CAD build for the part. Positions are in the model's coordinates, mm. Face numbers are marked on the shaded views. A direction names the side the tool comes from. Round coordinates to 2 decimals unless told otherwise and drop trailing zeros. Loops run counter-clockwise (first coordinate to the right, second up) from the corner with the lowest first, then second, coordinate; pieces in that order, holes last. Notation, with made-up numbers: (28.5, -6) -> (74.5, -6) arc R32 cw to (74.5, 26) -> close; hole circle Ø5 at (88, 38.25). An arc over 180 degrees is marked (long way). Answer as CSV lines item,"result".
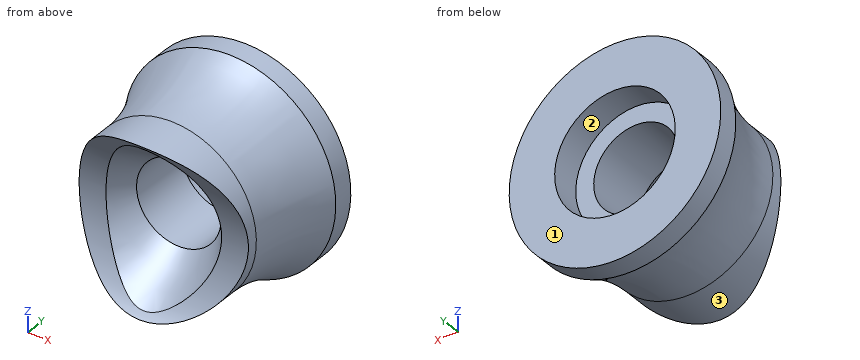
```python
from build123d import *

# Parameters (mm, degrees)
ENL_V_MAT_EXTRU_1_DEPTH      = 26
ENL_V_MAT_EXTRU_1_DEPTH_BACK = 26


with BuildPart() as part:
    # Esquisse1 → Révolution1 (revolve)
    with BuildSketch(Plane.XY, mode=Mode.PRIVATE) as r_volution1_sk:
        with BuildLine():
            Line((10, -22), (10, -7))
            Line((10, -7), (14.25, -7))
            Line((14.25, -7), (14.25, 0))
            Line((14.25, 0), (25, 0))
            Line((25, 0), (25, -5))
            ThreePointArc((25, -5), (21.270166538, -14.364916731), (20, -24.364916731))
            Line((20, -24.364916731), (20, -35))
            Line((20, -35), (19.5, -35))
            Line((19.5, -35), (10, -22))
        make_face()
    revolve(r_volution1_sk.sketch.rotate(Axis((0, 35.983333333, 0), (0, -1, 0)), 90), axis=Axis((0, 35.983333333, 0), (0, -1, 0)))  # turned: the seam where the file's is

    # Esquisse2 → Enlèv. mat.-Extru.1 (cut, two sides)
    with BuildSketch(Plane(origin=(0, 0, 0), x_dir=(0, 0, -1), z_dir=(1, 0, 0))) as enl_v_mat_extru_1_sk:
        with BuildLine():
            Line((109.805806645, -120.529339662), (20, -35))
            ThreePointArc((20, -35), (0, -27), (-20, -35))
            Line((-20, -35), (-109.805806645, -120.529339662))
            Line((-109.805806645, -120.529339662), (-109.805806645, -368.564424682))
            Line((-109.805806645, -368.564424682), (109.805806645, -368.564424682))
            Line((109.805806645, -368.564424682), (109.805806645, -120.529339662))
        make_face()
    extrude(amount=ENL_V_MAT_EXTRU_1_DEPTH, mode=Mode.SUBTRACT)
    extrude(enl_v_mat_extru_1_sk.sketch, amount=-ENL_V_MAT_EXTRU_1_DEPTH_BACK, mode=Mode.SUBTRACT)


solid = part.part
```
Q1. Slice it at D-D, the plane y = -14.5. Give the cut face in (x, z).
Results:
outline,"circle Ø42.47 at (0, 0); hole circle Ø20 at (0, 0)"
Q2. Tool access for the marked faces 1, 2 and 3: list every direction of +Z, -Z, +X, -X, +Y, -Y with a clear straight run to the whole face (end or side of a thin tool).
Results:
face 1,"+Z, -Z, +X, -X, +Y"
face 2,"+Y"
face 3,"-Y"
Q3. Slice it at B-B, the plane x = 0. Give the cut face in (y, z), and give its area (3 significant figures).
Results:
outline,"(-35, -20) -> (-24.36, -20) arc R40 cw to (-5, -25) -> (0, -25) -> (0, -14.25) -> (-7, -14.25) -> (-7, -10) -> (-22, -10) -> (-33.72, -18.57) arc R29 cw to start; (-35, 20) arc R29 cw to (-33.72, 18.57) -> (-22, 10) -> (-7, 10) -> (-7, 14.25) -> (0, 14.25) -> (0, 25) -> (-5, 25) arc R40 cw to (-24.36, 20) -> close"
area,"629 mm2"
Q4. Probe L1, parallel to X at y = -4.75, z = 0; L2, parallel to X at y = -13, z = 9; L3, parallel to Z at x = 7.5, y = -14. List the from-to ranges inside material, lowest first. Write a range as [from, to].
Results:
L1,"[-25, -14.25], [14.25, 25]"
L2,"[-19.69, -4.36], [4.36, 19.69]"
L3,"[-20.01, -6.61], [6.61, 20.01]"
Q5. Slice it at A-A, the plane z = 0. Give the cut face in (x, y).
Results:
outline,"(-25, -5) arc R40 cw to (-20, -24.36) -> (-20, -27) -> (-13.65, -27) -> (-10, -22) -> (-10, -7) -> (-14.25, -7) -> (-14.25, 0) -> (-25, 0) -> close; (10, -22) -> (13.65, -27) -> (20, -27) -> (20, -24.36) arc R40 cw to (25, -5) -> (25, 0) -> (14.25, 0) -> (14.25, -7) -> (10, -7) -> close"
Q6. Drop flat-ended pins along their axis: pin 1 Ø5 at (x, y) = (-7.5, -7) entering from +Z; pin 2 Ø12 at (y, z) = (-23.5, 19.5) entering from +X; pin 3 Ø14 at (x, z) = (-2, 6.5) entering from +Y; pin 4 Ø12 at (x, z) = (0, 0) entering from -Y. Give the stop position or say it passes through.
Results:
pin 1,"z = 24.27"
pin 2,"x = 14.77"
pin 3,"y = -7"
pin 4,"through"
Q7. Slice it at C-C, the plane y = -31. Give the cut face in (x, z).
Results:
outline,"(-13.56, -14.7) arc R20 ccw to (13.56, -14.7) -> (7.67, -14.7) arc R16.58 cw to (-7.67, -14.7) -> close; (-13.56, 14.7) -> (-7.67, 14.7) arc R16.58 cw to (7.67, 14.7) -> (13.56, 14.7) arc R20 ccw to start"
